For this review, use the dimensioned drawing (mm, ordinates from the lowest corner) and the shaded views. A direction names the side the tool comes from. Give positions to 0.01 mm unless a question says otherwise; leave off trailing zeros. Order: outer loops, then holes, each group sorted by start corner. A loop starts at its lowest first (then second) coordinate and runs counter-clockwise, first axis right, second up.
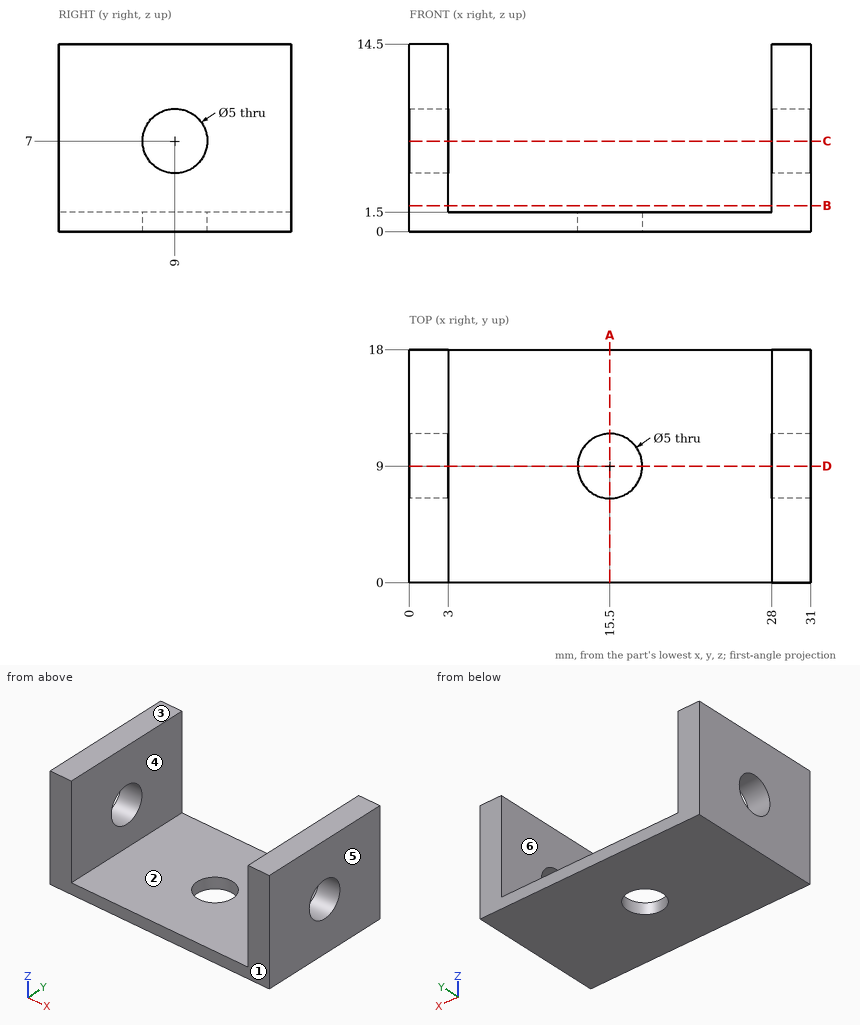
1. Take a section at D-D (y = 9). State the section outline as (x, z) points, then the cut area to 3 significant figures.
Recorded:
outline: (0, 0) - (13, 0) - (13, 1.5) - (3, 1.5) - (3, 4.5) - (0, 4.5) - close; (0, 9.5) - (3, 9.5) - (3, 14.5) - (0, 14.5) - close; (18, 0) - (31, 0) - (31, 4.5) - (28, 4.5) - (28, 1.5) - (18, 1.5) - close; (28, 9.5) - (31, 9.5) - (31, 14.5) - (28, 14.5) - close
area: 87.0 mm2
2. Take a section at A-A (x = 15.5). State the section outline as (y, z) points, then the cut area to 3 significant figures.
Recorded:
outline: (0, 0) - (6.5, 0) - (6.5, 1.5) - (0, 1.5) - close; (11.5, 0) - (18, 0) - (18, 1.5) - (11.5, 1.5) - close
area: 19.5 mm2
3. Take a section at B-B (z = 2). State the section outline as (x, y) points, then the cut area to 3 significant figures.
Recorded:
outline: (0, 0) - (3, 0) - (3, 18) - (0, 18) - close; (28, 0) - (31, 0) - (31, 18) - (28, 18) - close
area: 108 mm2
4. Draft analysis for pull direction X (two halves, no side actions). For the marked faces 3, 4, 5 and 6, state which applies: pulls with the +X half, pulls with the -X half, needs draft (parallel to the pull), parting line crosses it, or undercut.
Recorded:
face 3: needs draft
face 4: undercut
face 5: pulls with the +X half
face 6: undercut
5. For pin 1 (1 mm diameter, centred on x = 12, y = 10.5, fed in from +Z), flat-tipped, find the tip position at first contact; note if it passes through.
Recorded:
pin 1: stops at z = 1.5
6. For line 1 along X through (y, z) = (4.25, 1.75); line 2 along Y through (x, z) = (15.5, 0.75); line 3 along Z through (x, y) = (22.5, 10.5), list the stretches that pass through material, from the lowest coordinate up.
Recorded:
line 1: x = 0 to 3, 28 to 31
line 2: y = 0 to 6.5, 11.5 to 18
line 3: z = 0 to 1.5
7. Take a section at C-C (z = 7). State the section outline as (x, y) points, then the cut area to 3 significant figures.
Recorded:
outline: (0, 0) - (3, 0) - (3, 6.5) - (0, 6.5) - close; (0, 11.5) - (3, 11.5) - (3, 18) - (0, 18) - close; (28, 0) - (31, 0) - (31, 6.5) - (28, 6.5) - close; (28, 11.5) - (31, 11.5) - (31, 18) - (28, 18) - close
area: 78.0 mm2
8. Machinability: for the marked faces 1 and 2, which of the approach directions +Z, -Z, +X, -X, +Y, -Y give a long, thin tool a straight path to every point of the face, cutting with its end or side? Answer none if there is none.
Recorded:
face 1: +Z, -Z, +X, -X, -Y
face 2: +Z, +Y, -Y
